```python
from build123d import *

# Parameters (mm, degrees)
F1_DEPTH = 60
F2_DEPTH = 30
F3_DEPTH = 12.5
F5_R     = 10


# Not quite as in the source:
# - a feature names something its author has since deleted; it is built from what else it names


with BuildPart() as f1:
    # F0 (on Front) → F1 (new body, symmetric)
    with BuildSketch(Plane.XZ):
        Polygon((-60, 12.5), (-60, -12.5), (60, -12.5), (60, 12.5), (38, 12.5), align=None)
    extrude(amount=F1_DEPTH, both=True)

    # F0 (on Front) → F2 (join, symmetric)
    with BuildSketch(Plane.XZ):
        with BuildLine():
            Line((38, 12.5), (60, 12.5))
            Line((60, 12.5), (60, 27.5))
            ThreePointArc((60, 27.5), (64.1886116992, 39.7474487139), (75, 46.864916731))
            Line((75, 46.864916731), (75, 69.1849707307))
            add(Edge.make_bspline(
                [(74.6086884092, 69.1525360492), (74.7393390429, 69.163538875), (74.8697772932, 69.1743509337), (75, 69.1849707307)],
                knots=[0.9728827871, 0.9728827871, 0.9728827871, 0.9728827871, 0.9748058763, 0.9748058763, 0.9748058763, 0.9748058763], degree=3))
            ThreePointArc((74.6086884092, 69.1525360492), (48.4529313025, 55.2269265623), (38, 27.5))
            Line((38, 27.5), (38, 12.5))
        make_face()
        with BuildLine():
            ThreePointArc((80, 69.5), (77.4955434529, 69.425263236), (75, 69.201318924))
            Line((75, 69.201318924), (75, 69.1849707307))
            add(Edge.make_bspline(
                [(75, 69.1849707307), (76.7060295657, 69.324099213), (78.3750648422, 69.4302293108), (80, 69.5)],
                knots=[0.9748058763, 0.9748058763, 0.9748058763, 0.9748058763, 1, 1, 1, 1], degree=3))
        make_face()
        with BuildLine():
            add(Edge.make_bspline(
                [(75, 69.1849707307), (76.7060295657, 69.324099213), (78.3750648422, 69.4302293108), (80, 69.5)],
                knots=[0.9748058763, 0.9748058763, 0.9748058763, 0.9748058763, 1, 1, 1, 1], degree=3))
            Line((75, 69.1849707307), (75, 46.864916731))
            ThreePointArc((75, 46.864916731), (77.4799141503, 47.3405939253), (80, 47.5))
            Line((80, 47.5), (105, 47.5))
            Line((105, 47.5), (105, 69.5))
            Line((105, 69.5), (80, 69.5))
        make_face()
    extrude(amount=F2_DEPTH, both=True)

    # F0 (on Front) → F3 (join, symmetric)
    with BuildSketch(Plane.XZ):
        with BuildLine():
            add(Edge.make_bspline(
                [(-60, 12.5), (-58.7895740645, 37.710647482), (-15.7147551824, 47.8502400891), (-15.7294783827, 47.857399648), (37.8509932243, 66.056963491), (74.6086884092, 69.1525360492)],
                knots=[0, 0, 0, 0, 0.4317155285, 0.4318343159, 0.9728827871, 0.9728827871, 0.9728827871, 0.9728827871], degree=3))
            Line((-60, 12.5), (38, 12.5))
            Line((38, 12.5), (38, 27.5))
            ThreePointArc((38, 27.5), (48.4529313025, 55.2269265623), (74.6086884092, 69.1525360492))
        make_face()
    extrude(amount=F3_DEPTH, both=True)

    # F0 (on Front) → F4 (revolve)
    with BuildSketch(Plane.XZ):
        Polygon((135, 72.5), (105, 72.5), (105, 69.5), (105, 47.5), (105, 42.5), (135, 42.5), align=None)
    revolve(axis=Axis((105, 0, 58.5), (0, 0, 1)))

    # F5
    f5_edges = [f1.edges().sort_by_distance(p)[0] for p in [
        (-60, -60, 0),
        (60, -60, 0),
        (60, 60, 0),
        (-60, 60, 0),
    ]]
    fillet(f5_edges, radius=F5_R)


solid = f1.part
```
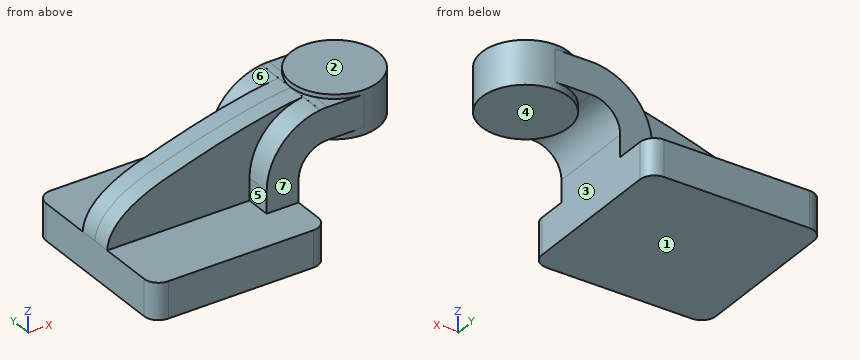
Check sheet for the modelled part. Datum: model origin and axes. Units: mm. Face numbers are marked on the shaded views. A direction names the side the tool comes from. Coordinates: 2 decimals unless noted, no trailing zeros. Loops run counter-clockwise (first coordinate to the right, second up) from the corner with the lowest first, then second, coordinate; pieces in that order, holes last.
1) Material ranges on probe 1 along Z at (x, y) = (-40, 28.5); probe 2 along Y at (x, z) = (40, 20.5); probe 3 along X at (y, z) = (-49, 6), recorded low to high.
2) Sectioned sample at A-A (x = 121). Record the boundary of the cut face in (y, z).
3) Release check for a two-part mould opening along Z. For the marked faces 1, 2 and 3 record: released by +Z, released by -Z, zero draft, split by the parting line, or undercut.
4) Access from +Z, -Z, +X, -X, +Y, -Y to the whole of each face (thin tool, end or side, straight path). Record for the marked faces 4, 5, 6 and 7.
5) Gauge pin test, flat ends, axial feed: pin 1 (10.5 mm diameter, centred on x = 88, y = -22.5, fed in from -Z); pin 2 (3 mm diameter, centred on y = -4.5, z = 20, fed in from +X); pin 3 (2 mm diameter, centred on x = 28.5, z = 55, fed in from -Y). Record the tip position at first contact, or that the pin passes through.
Check sheet entries:
1. probe 1: z = -12.5 to 12.5
1. probe 2: y = -30 to 30
1. probe 3: x = -60 to 60
2. outline: (-25.38, 42.5) - (25.38, 42.5) - (25.38, 72.5) - (-25.38, 72.5) - close
3. face 1: released by -Z
3. face 2: released by +Z
3. face 3: zero draft
4. face 4: -Z, +X, +Y, -Y
4. face 5: +Z, -X, -Y
4. face 6: +Z, -X, +Y
4. face 7: +Z, +X, -X, -Y
5. pin 1: stops at z = 42.5
5. pin 2: stops at x = 60
5. pin 3: stops at y = -12.5
